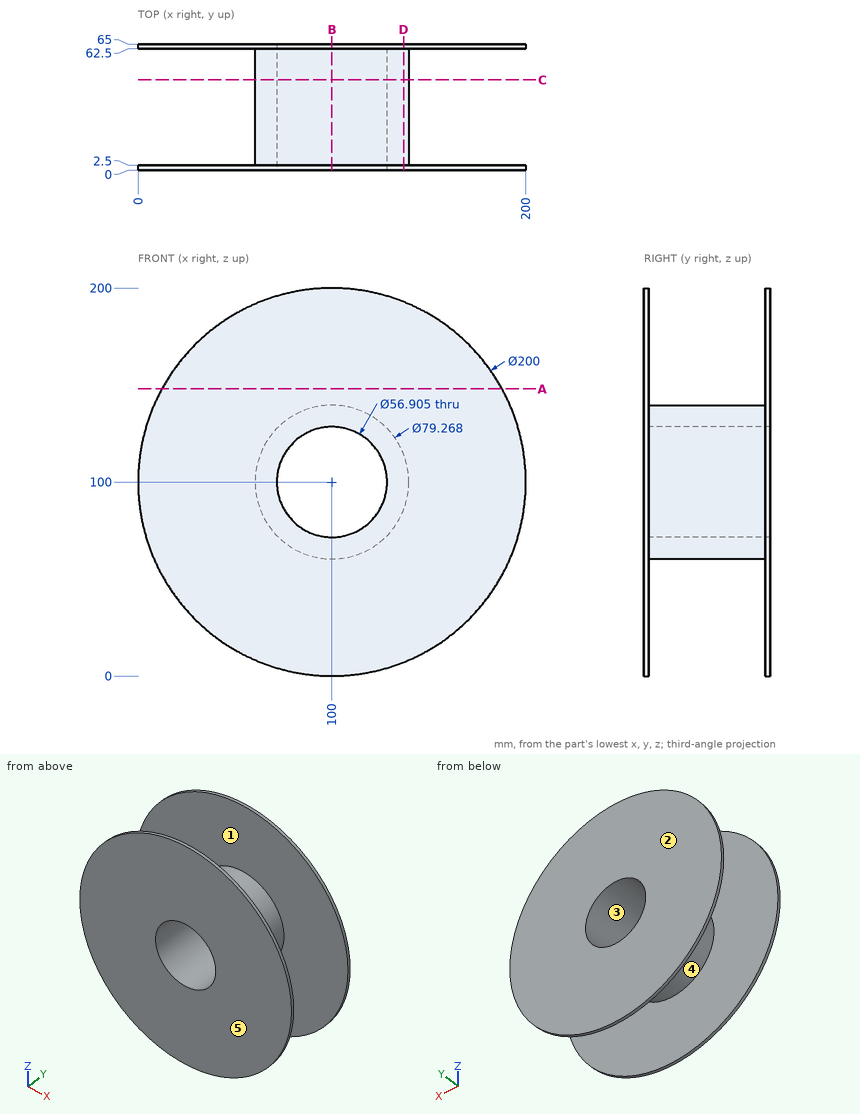
Print and shaded views of the part. All mm, measured from the part's lowest x, y and z. A direction names the side the tool comes from. Give positions to 0.01 mm unless a question says otherwise; leave off trailing zeros. Order: outer loops, then holes, each group sorted by start corner. A loop starts at its lowest first (then second) coordinate and runs counter-clockwise, first axis right, second up. Notation, with made-up numbers: (-34, 21) -> (15, 21) arc R11 cw to (15, 33) -> close; hole circle Ø2 at (-32, 52.5). An arc over 180 degrees is marked (long way). Use CSV: the item, a comma, the result in double quotes.
1. Band-saw the part on A-A, the plane z = 148. Give the cut face in (x, y), then the cut area to 3 significant figures.
Outcome:
outline,"(12.27, 0) -> (187.73, 0) -> (187.73, 2.5) -> (12.27, 2.5) -> close; (12.27, 62.5) -> (187.73, 62.5) -> (187.73, 65) -> (12.27, 65) -> close"
area,"877 mm²"
2. Band-saw the part on B-B, the plane x = 100. Give the cut face in (y, z), then the cut area to 3 significant figures.
Outcome:
outline,"(0, 0) -> (2.5, 0) -> (2.5, 60.37) -> (62.5, 60.37) -> (62.5, 0) -> (65, 0) -> (65, 71.55) -> (0, 71.55) -> close; (0, 128.45) -> (65, 128.45) -> (65, 200) -> (62.5, 200) -> (62.5, 139.63) -> (2.5, 139.63) -> (2.5, 200) -> (0, 200) -> close"
area,"2,060 mm²"
3. 3-axis set-ups, long thin cutter, end or side, ignore diameter. For the marked faces 1 and 2: which of +Z, -Z, +X, -X, +Y, -Y reach the whole face in a straight line?
Outcome:
face 1,"none"
face 2,"+Z, -Z, +X, -X, +Y"
4. Mould opens along Z. For the marked faces 3, 4 and 5 say: +Z half, -Z half, draft (parallel to the pull), parting line (faces both ways), or undercut.
Outcome:
face 3,"undercut"
face 4,"parting line"
face 5,"draft"
5. Drill centre lines: line 1 along Y through (x, z) = (177.5, 120); line 2 along Z through (x, y) = (100, 29.5); line 3 along Z through (x, y) = (87, 46). Where is each one in solid material? Low to high. Write a range as from..to.
Outcome:
line 1,"0..2.5, 62.5..65"
line 2,"60.37..71.55, 128.45..139.63"
line 3,"62.56..74.69, 125.31..137.44"
6. Drop flat-ended pins along their axis: pin 1 (5 mm diameter, centred on y = 14, z = 133.5, fed in from -X) (1 decimal); pin 2 (1 mm diameter, centred on x = 137, y = 21, fed in from +Z); pin 3 (4 mm diameter, centred on x = 126, y = 34, fed in from +Z). Give the stop position or say it passes through.
Outcome:
pin 1,"x = 75.3"
pin 2,"z = 115.45"
pin 3,"z = 131.54"
7. Band-saw the part on C-C, the plane y = 46.5. Give the cut face in (x, z) (1 decimal), then the cut area to 3 significant figures.
Outcome:
outline,"circle Ø79.3 at (100, 100); hole circle Ø56.9 at (100, 100)"
area,"2,390 mm²"
8. Band-saw the part on D-D, the plane x = 137. Give the cut face in (y, z), then the cut area to 3 significant figures.
Outcome:
outline,"(0, 7.1) -> (2.5, 7.1) -> (2.5, 85.79) -> (62.5, 85.79) -> (62.5, 7.1) -> (65, 7.1) -> (65, 192.9) -> (62.5, 192.9) -> (62.5, 114.21) -> (2.5, 114.21) -> (2.5, 192.9) -> (0, 192.9) -> close"
area,"2,630 mm²"
